Autodesk Inventor part; units mm, degrees
ref_plane "YZ Plane" through (0, 0, 0) normal (1, 0, 0) x (0, 1, 0)
ref_plane "XZ Plane" through (0, 0, 0) normal (0, 1, 0) x (-1, 0, 0)
ref_plane "XY Plane" through (0, 0, 0) normal (0, 0, 1) x (1, 0, 0)
sketch "Sketch1" plane through (0, 0, 0) normal (0, 1, 0) x (-1, 0, 0)
  line L0 (101.6, 6.35) -> (-101.6, 6.35)
  line L1 (-101.6, -6.35) -> (101.6, -6.35)
  arc A0 (101.6, -6.35) -> (101.6, 6.35) centre (101.6, 0) ccw
  arc A1 (-101.6, 6.35) -> (-101.6, -6.35) centre (-101.6, 0) ccw
  line L2 (151.13, 0) -> (-151.13, 0)
  line L3 (0, -8.89) -> (0, 8.89)
  point P0 (0, 0)
  dimension "d2" = 203.2
  dimension "d3" = 6.35
  dimension "d4" = 6.35
  dimension "d5" = 101.6
  dimension "d6" = 0
  dimension "d7" = 12.7
  dimension "d9" = 6.35
  dimension "d37" = 203.2
extrude "Extrusion1" add sketch "Sketch1" along normal blind 12.7
sketch "Sketch4" plane through (0, 12.7, 0) normal (0, 1, 0) x (1, 0, 0)
  circle A0 centre (-101.6, 0) radius 3.175
  line L0 (-151.13, 0) -> (151.13, 0)
  line L1 (0, 8.89) -> (0, -8.89)
  circle A1 centre (-76.2, 0) radius 3.175
  circle A2 centre (-50.8, 0) radius 3.175
  circle A3 centre (-25.4, 0) radius 3.175
  circle A4 centre (0, 0) radius 3.175
  circle A5 centre (25.4, 0) radius 3.175
  circle A6 centre (50.8, 0) radius 3.175
  circle A7 centre (76.2, 0) radius 3.175
  circle A8 centre (101.6, 0) radius 3.175
  dimension "d45" = 6.35
  dimension "d46" = 101.6
  dimension "d47" = 0
  dimension "d50" = 25.4
extrude "Extrusion4" cut sketch "Sketch4" against normal through all
sketch "Sketch5" plane through (0, 12.7, 0) normal (0, 1, 0) x (1, 0, 0)
  line L0 (-95.25, -3.175) -> (-82.55, -3.175)
  line L1 (-82.55, -3.175) -> (-82.55, 3.175)
  line L2 (-82.55, 3.175) -> (-95.25, 3.175)
  line L3 (-95.25, 3.175) -> (-95.25, -3.175)
  line L4 (-151.13, 0) -> (151.13, 0)
  line L5 (0, 13.6448) -> (0, -37.419)
  line L6 (-57.15, 3.175) -> (-69.85, 3.175)
  line L7 (-69.85, 3.175) -> (-69.85, -3.175)
  line L8 (-69.85, -3.175) -> (-57.15, -3.175)
  line L9 (-57.15, -3.175) -> (-57.15, 3.175)
  line L10 (-31.75, 3.175) -> (-44.45, 3.175)
  line L11 (-44.45, 3.175) -> (-44.45, -3.175)
  line L12 (-44.45, -3.175) -> (-31.75, -3.175)
  line L13 (-31.75, -3.175) -> (-31.75, 3.175)
  line L14 (-6.35, 3.175) -> (-19.05, 3.175)
  line L15 (-19.05, 3.175) -> (-19.05, -3.175)
  line L16 (-19.05, -3.175) -> (-6.35, -3.175)
  line L17 (-6.35, -3.175) -> (-6.35, 3.175)
  line L18 (19.05, 3.175) -> (6.35, 3.175)
  line L19 (6.35, 3.175) -> (6.35, -3.175)
  line L20 (6.35, -3.175) -> (19.05, -3.175)
  line L21 (19.05, -3.175) -> (19.05, 3.175)
  line L22 (44.45, 3.175) -> (31.75, 3.175)
  line L23 (31.75, 3.175) -> (31.75, -3.175)
  line L24 (31.75, -3.175) -> (44.45, -3.175)
  line L25 (44.45, -3.175) -> (44.45, 3.175)
  line L26 (69.85, 3.175) -> (57.15, 3.175)
  line L27 (57.15, 3.175) -> (57.15, -3.175)
  line L28 (57.15, -3.175) -> (69.85, -3.175)
  line L29 (69.85, -3.175) -> (69.85, 3.175)
  line L30 (95.25, 3.175) -> (82.55, 3.175)
  line L31 (82.55, 3.175) -> (82.55, -3.175)
  line L32 (82.55, -3.175) -> (95.25, -3.175)
  line L33 (95.25, -3.175) -> (95.25, 3.175)
  point P0 (0, 0)
  dimension "d57" = 12.7
  dimension "d58" = 6.35
  dimension "d59" = 82.55
  dimension "d60" = 3.175
  dimension "d63" = 25.4
extrude "Extrusion5" cut sketch "Sketch5" against normal through all
properties part number "8M Module" material "Wood (Cherry)"
Here's how the part is built. I have some questions about the finished solid (model axes, mm). Give positions to 0.01 mm unless a question says otherwise; leave off trailing zeros. Loops run counter-clockwise (first coordinate to the right, second up) from the corner with the lowest first, then second, coordinate; pieces in that order, holes last. Notation, with made-up numbers: (22.5, 86.25) -> (66.5, 86.25) arc R21 ccw to (66.5, 118.25) -> close; hole circle Ø1 at (73.25, 53). An arc over 180 degrees is marked (long way). Answer as a JSON object with one key per item and string values. Group by question number.
Item 1: Imagine slicing it at B-B on y = 7.75. Give the number of separate pieces and of enclosed holes in the cut face, then the cut area to 3 significant figures.
Item 2: Thinking about a two-plate mould opening in X: for faces 1 (the flat face through (-1, 6, 6.35)), 2 (the flat face through (31.75, 6, 0)), 3 (the cylindrical face through (-107.95, 6.26, 0.14)), which applies, pulls with the +X half, pulls with the -X half, needs draft (parallel to the pull), parting line crosses it, or undercut?
Item 3: Imagine slicing it at A-A on x = -76.2. Write out the boundary of the cut face in (y, z) (3 decimals).
Item 4: Will these pins go through, and if not, where does the flat tip stop? pin 1 (1.5 mm diameter, centred on y = 7.5, z = -5, fed in from -X); pin 2 (1.9 mm diameter, centred on y = 5, z = -1, fed in from -X); pin 3 (5 mm diameter, centred on y = 8, z = -4.5, fed in from -X).
Item 5: I need wall thicknesses on L1, parallel to Z at x = 40, y = 1.75 (3 decimals); L2, parallel to X at y = 4, z = 3.25; L3, parallel to X at y = 6.5, z = 4.5. Which ranges of each line are inside material? Lowest first, please.
Answer list:
{
 "1": {"separate pieces": "1", "enclosed holes": "17", "area": "1,780 mm2"},
 "2": {"face 1": "needs draft", "face 2": "undercut", "face 3": "pulls with the -X half"},
 "3": {"outline": "(0, -6.35) -> (12.7, -6.35) -> (12.7, -3.175) -> (0, -3.175) -> close; (0, 3.175) -> (12.7, 3.175) -> (12.7, 6.35) -> (0, 6.35) -> close"},
 "4": {"pin 1": "stops at x = -106.32", "pin 2": "stops at x = -107.95", "pin 3": "stops at x = -107.63"},
 "5": {"L1": "z = -6.35 to -3.175, 3.175 to 6.35", "L2": "x = -107.06 to 107.06", "L3": "x = -106.08 to 106.08"}
}
